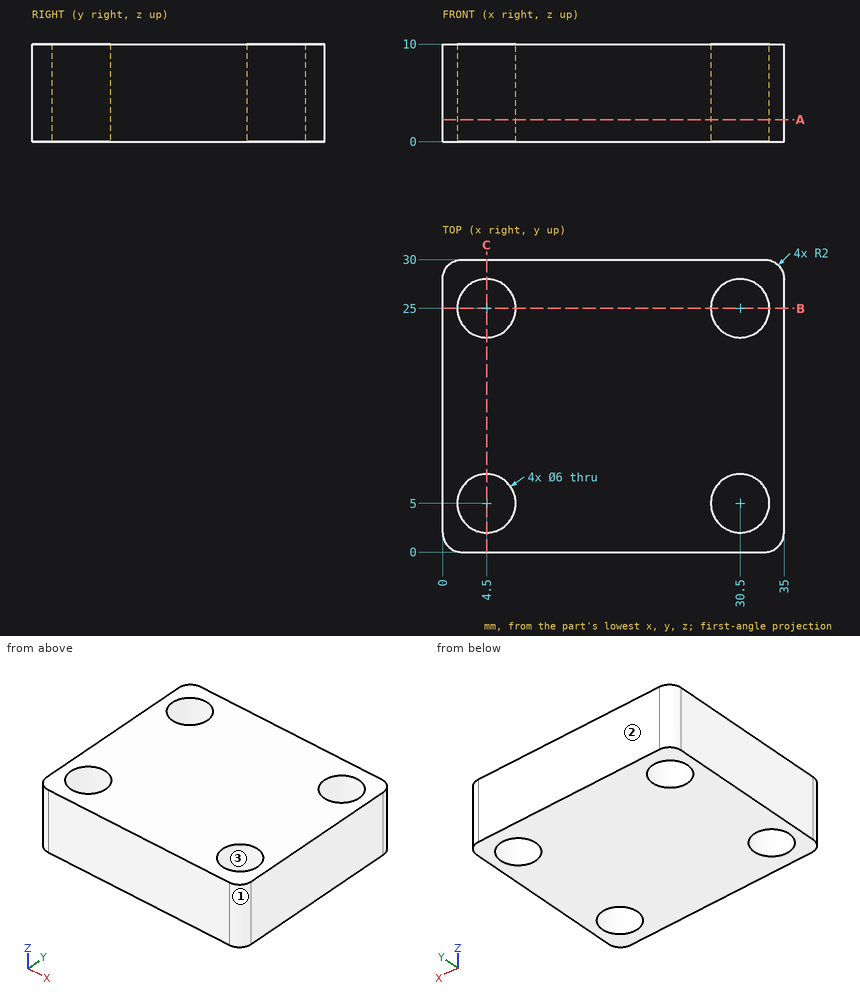
Geometry: see drawing. Coordinates: mm, zero at the bounding-box minimum. Give positions to 0.01 mm unless a question says otherwise; leave off trailing zeros. Loops run counter-clockwise (first coordinate to the right, second up) from the corner with the lowest first, then second, coordinate; pieces in that order, holes last. Notation, with made-up numbers: (18, -3.5) - (47, -3.5) arc R27 ccw to (47, 22.5) - close; hole circle Ø4 at (-8, -37). An arc over 180 degrees is marked (long way). Use CSV: the item, a comma, the result in double quotes. Start each with the question number.
Item 1: Section C-C on x = 4.5. Return loops of the section in (y, z).
Item 2: Contact query for a flat-ended pin moving along its axis: P1, Ø5, axis at x = 4.5, y = 25, coming from the +Z side. Output: stop coordinate, or through.
Item 3: Mould query, pull axis Y, two halves, no side actions, for the marked faces 1, 2 and 3. Classes: pulls with the +Y half, pulls with the -Y half, needs draft (parallel to the pull), parting line crosses it, or undercut.
Item 4: Section A-A on z = 2.25. Return loops of the section in (x, y), then the cut area to 3 significant figures.
Item 5: Line query: line 1 (Y direction, x = 4.5, z = 3.75); line 2 (X direction, y = 3.75, z = 7.5); line 3 (Y direction, x = 3, z = 2.5). Output: solid intervals per line, ascending.
Item 6: Section B-B on y = 25. Return loops of the section in (x, z), then the cut area to 3 significant figures.
Ans:
1,outline,"(0, 0) - (2, 0) - (2, 10) - (0, 10) - close; (8, 0) - (22, 0) - (22, 10) - (8, 10) - close; (28, 0) - (30, 0) - (30, 10) - (28, 10) - close"
2,P1,"passes through"
3,face 1,"pulls with the -Y half"
3,face 2,"pulls with the +Y half"
3,face 3,"undercut"
4,outline,"(0, 2) arc R2 ccw to (2, 0) - (33, 0) arc R2 ccw to (35, 2) - (35, 28) arc R2 ccw to (33, 30) - (2, 30) arc R2 ccw to (0, 28) - close; hole circle Ø6 at (4.5, 5); hole circle Ø6 at (4.5, 25); hole circle Ø6 at (30.5, 5); hole circle Ø6 at (30.5, 25)"
4,area,"933 mm2"
5,line 1,"y = 0 to 2, 8 to 22, 28 to 30"
5,line 2,"x = 0 to 1.77, 7.23 to 27.77, 33.23 to 35"
5,line 3,"y = 0 to 2.4, 7.6 to 22.4, 27.6 to 30"
6,outline,"(0, 0) - (1.5, 0) - (1.5, 10) - (0, 10) - close; (7.5, 0) - (27.5, 0) - (27.5, 10) - (7.5, 10) - close; (33.5, 0) - (35, 0) - (35, 10) - (33.5, 10) - close"
6,area,"230 mm2"
